Input: dimensioned drawing with shaded views. Units: mm. Origin: part minimum x, y, z. A direction names the side the tool comes from. Give positions to 0.01 mm unless a question says otherwise; leave off trailing zeros. Order: outer loops, then holes, each group sorted by start corner. A loop starts at its lowest first (then second) coordinate and runs counter-clockwise, first axis right, second up.
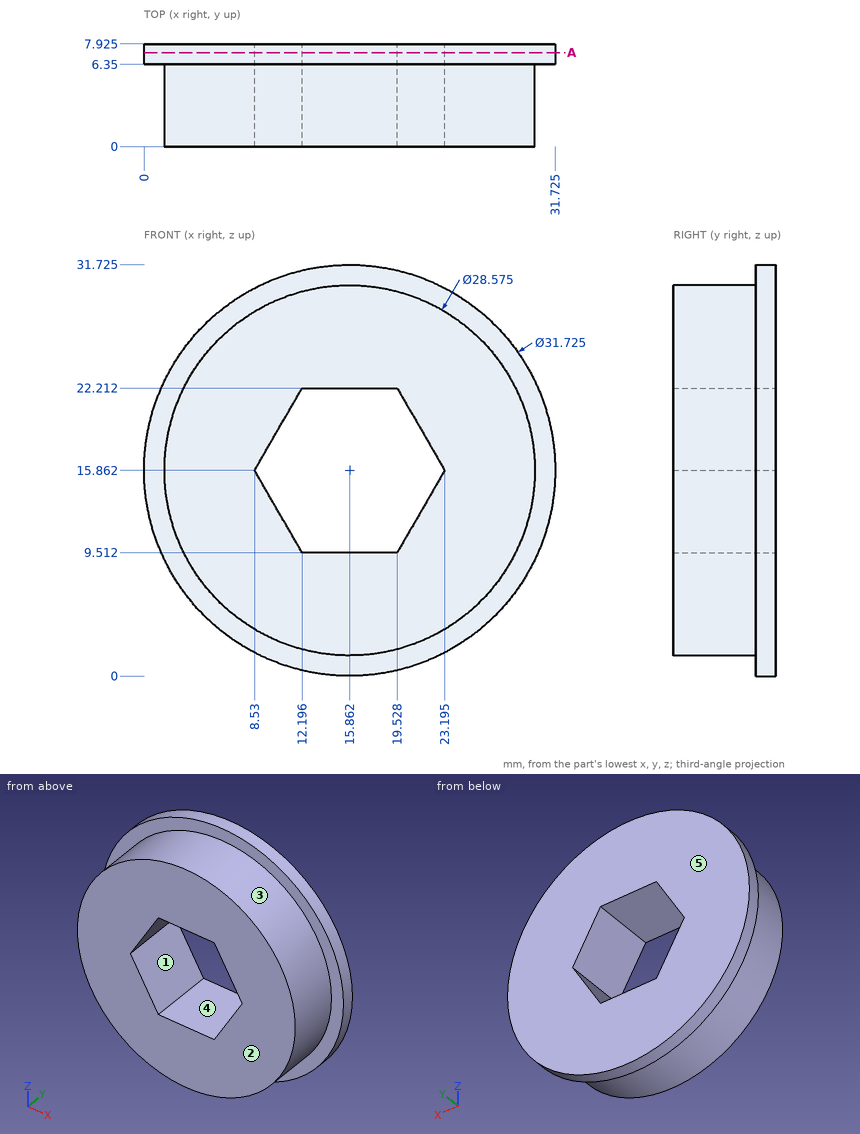
1) Draft query along Z for the marked faces 3, 4 and 5. Return one class per face: +Z half, -Z half, draft (parallel to the pull), parting line (faces both ways), or undercut.
Report:
face 3: parting line
face 4: undercut
face 5: draft
2) Material intervals for L1, parallel to Z at x = 10, y = 1 (1 decimal); L2, parallel to X at y = 5.5, z = 15.5 (1 decimal); L3, parallel to Z at x = 11, y = 4.25 (1 decimal), sorted ascending.
Report:
L1: z = 2.8 to 13.3, 18.4 to 28.9
L2: x = 1.6 to 8.7, 23 to 30.1
L3: z = 2.4 to 11.6, 20.1 to 29.3
3) Reachability of the marked faces 1 and 2 from +Z, -Z, +X, -X, +Y, -Y: full face, straight path, thin tool, end or side. Return the list, or none.
Report:
face 1: +Y, -Y
face 2: +Z, -Z, +X, -X, -Y
4) Section query A-A, the plane y = 7.25. Return the cut outline in (x, z) (1 decimal), and give its area (3 significant figures).
Report:
outline: circle Ø31.7 at (15.9, 15.9); hole (8.5, 15.9) - (12.2, 9.5) - (19.5, 9.5) - (23.2, 15.9) - (19.5, 22.2) - (12.2, 22.2) - close
area: 651 mm2
5) Pin query (flat end, axial travel): pin 1 (4 mm diameter, centred on y = 5.5, z = 27, fed in from -X); pin 2 (4 mm diameter, centred on x = 14, z = 13, fed in from -Y); pin 3 (3.5 mm diameter, centred on x = 17, y = 3, fed in from +Z). Return the tip coordinate at first contact, or that it passes through.
Report:
pin 1: stops at x = 3.03
pin 2: passes through
pin 3: stops at z = 30.15
